Could you check a few things on this model? Use its own coordinates, in mm. A direction names the side the tool comes from. Round coordinates to 2 decimals unless told otherwise and drop trailing zeros. Write each loop counter-clockwise with the first axis right and the second up, starting at its lowest first coordinate (ties: lowest second). Pieces come first, ordered by that corner, then holes. Notation, with made-up numbers: M 64,34.25 L 122,34.25 A37 cw 122,72.25 Z; hole C 56.25,87.5 d11. An arc over 180 degrees is marked long. One line per question, with ' | ' between items. Start each with the question number.
Autodesk Fusion 360 part; units mm, degrees
sketch "Sketch1" plane through (0, 0, 0) normal (0, 1, 0) x (1, 0, 0)
  circle A0 centre (0, 0) radius 2.75
  circle A1 centre (0, 0) radius 6.75
  dimension "d1" = 5.5
  dimension "d2" = 4
extrude "Extrude1" add sketch "Sketch1" along normal blind 12
ref_plane "WorkPlane1" through (3, 0, 0) normal (1, 0, 0) x (0, 1, 0)
sketch "Sketch2" plane through (3, 0, 0) normal (1, 0, 0) x (0, 1, 0)
  line L0 (12, -6.75) -> (12, 6.75)
  line L1 (0, -6.75) -> (0, 6.75)
  circle A0 centre (6, 0) radius 4.6
  circle A1 centre (6, 0) radius 6
  dimension "d6" = 9.2
  dimension "d7" = 6
  dimension "d8" = 12
  dimension "d9" = 1.4
extrude "Extrude2" add sketch "Sketch2" along normal blind 8
ref_plane "WorkPlane2" through (2.75, 6.403, 0) normal (-1, 0, 0) x (0, 0, -1)
sketch "Sketch3" plane through (2.75, 6.403, 0) normal (-1, 0, 0) x (0, -1, 0)
  line L0 (-5.597, -2.75) -> (-5.597, 2.75)
  line L1 (6.403, -2.75) -> (6.403, 2.75)
  line L2 (6.403, -2.75) -> (6.403, 2.75)
  line L3 (-5.597, -2.75) -> (-5.597, 2.75)
  circle A0 centre (0.403, 0) radius 3.5
  point P0 (0.403, 0)
  dimension "d13" = 6
  dimension "d14" = 12
  dimension "d20" = 7
hole "Hole1" at (2.75, 6, 0) direction (1, 0, 0) diameter 3 depth 10 tip angle 118 counterbore diameter 7 counterbore depth 2
extrude "Extrude3" cut sketch "Sketch3" along normal blind 14.5
equation "d1 = 5 mm + 0.5 mm"
equation "d6 = 9 mm + 0.2 mm"
equation "d7 = d8 / 2"
equation "d13 = d14 / 2"
1. If we mould it in two halves opening along Y, with no side actions, what happens to faces 5 (the face through (3, 0, 0)), 6 (the face through (6.75, 7.98, -0.07)), 7 (the face through (7.869, 4.699, 5.857))? For each: released by +Y, released by -Y, zero draft, split by the parting line, or undercut.
2. I need wall thicknesses on line 1 along X through (y, z) = (1.9, 0); line 2 along Y through (x, z) = (-3.5, 0); line 3 along Z through (x, y) = (7, 6). Which ranges of each line are inside material? Lowest first, please. Write a range as from..to.
3. Suppose I cut it at A-A (x = 0). Write out the boundary of the cut face in (y, z).
4. Suppose I cut it at C-C (x = 8.5). Write out the boundary of the cut face in (y, z).
5. Suppose I cut it at D-D (y = 6.25). Write out the boundary of the cut face in (x, z), and give its area (3 significant figures).
6. I'm going to push flat-ended pins straight in: P1, Ø2, axis at x = -4.5, y = 2, coming from the +Z side; P2, Ø1, axis at y = 9, z = 1.5, coming from the +X side; P3, Ø2, axis at y = 5.5, z = 0.5, coming from the -X side; P4, Ø4.5, axis at x = 0, z = 0, coming from the -Y side. Where does each tip first touch, or does it pass through?
7. Which directions (+Z, -Z, +X, -X, +Y, -Y) give clear straight access to the entire face, cutting with the end or side of a thin tool? Please do faces 1 (the face through (-5.357, 5.916, -4.107)), 2 (the face through (11, 9, -4)), 3 (the face through (8.601, 8.123, 4.081)), 4 (the face through (4.75, 8, 0)).
Computed:
1) face 5: released by -Y | face 6: undercut | face 7: split by the parting line
2) line 1: x = -6.75..-2.75, 2.75..6.75 | line 2: y = 0..2.5, 9.5..12 | line 3: z = -6..-4.6, 4.6..6
3) outline: M 0,-6.75 L 12,-6.75 L 12,-2.75 L 8.17,-2.75 A3.5 cw 3.83,-2.75 L 0,-2.75 Z; M 0,2.75 L 3.83,2.75 A3.5 cw 8.17,2.75 L 12,2.75 L 12,6.75 L 0,6.75 Z
4) outline: C 6,0 d12; hole C 6,0 d9.2
5) outline: M -5.78,-3.49 A6.75 ccw 3.1,-5.99 L 11,-5.99 L 11,-4.59 L 4.95,-4.59 A6.75 ccw 6.59,-1.48 L 4.75,-1.48 L 4.75,-3.49 Z; M -5.78,3.49 L 4.75,3.49 L 4.75,1.48 L 6.59,1.48 A6.75 ccw 4.95,4.59 L 11,4.59 L 11,5.99 L 3.1,5.99 A6.75 ccw Z | area: 78.5 mm²
6) P1: stops at z = 5.77 | P2: stops at x = 6.68 | P3: stops at x = 4.75 | P4: passes through
7) face 1: none | face 2: +Z, -Z, +X, +Y, -Y | face 3: +X | face 4: -X
